Autodesk Fusion 360 part; units mm, degrees
sketch "Sketch1" plane through (0, 0, 0) normal (1, 0, 0) x (0, 1, 0)
  line L0 (0, 0) -> (101.6, 0)
  line L1 (101.6, 0) -> (101.6, 381)
  line L2 (101.6, 381) -> (0, 381)
  line L3 (0, 381) -> (0, 0)
  line L4 (50.8, 381) -> (0, 381)
  line L5 (0, 381) -> (0, 374.65)
  line L6 (0, 374.65) -> (50.8, 374.65)
  line L7 (50.8, 374.65) -> (50.8, 381)
  dimension "d1" = 101.6
  dimension "d2" = 381
  dimension "d3" = 6.35
  dimension "d5" = 50.8
extrude "Extrude1" add sketch "Sketch1" along normal blind 6.35 contours L0 L1 L2 L3 L6 L7
Can you work these out from the model? Positions are in its coordinate system, mm. A direction names the side the tool comes from. Coordinates: 2 decimals unless noted, no trailing zeros. Loops run counter-clockwise (first coordinate to the right, second up) from the corner with the lowest first, then second, coordinate; pieces in that order, holes last. Notation, with made-up numbers: (40, -32.5) - (81, -32.5) arc R27 cw to (81, -16.5) - close; hole circle Ø2 at (-27, -19). An arc over 180 degrees is marked (long way). Answer as CSV lines item,"result". Start each with the question number.
1) Which directions (+Z, -Z, +X, -X, +Y, -Y) give clear straight access to the entire face, cutting with the end or side of a thin tool? Please do faces 1 (the flat face through (3, 50, 0)), 2 (the flat face through (3, 25, 374.65)).
2) For pin 1 (1.9 mm diameter, centred on x = 2.5, y = 20, fed in from +Z); pin 2 (3 mm diameter, centred on x = 2.5, z = 378.5, fed in from -Y), each with a flat end and sliding along its axis, tell me the tip position at first contact or that it passes through.
3) I need wall thicknesses on line 1 (Z direction, x = 5.25, y = 31.5). Which ranges of the line are inside material? Lowest first, please. Write a range as from..to.
4) Suppose I cut it at A-A (y = 19). Please give me the cut outline in (x, z).
Check result:
1,face 1,"-Z, +X, -X, +Y, -Y"
1,face 2,"+Z, +X, -X, -Y"
2,pin 1,"stops at z = 374.65"
2,pin 2,"stops at y = 50.8"
3,line 1,"z = 0..374.65"
4,outline,"(0, 0) - (6.35, 0) - (6.35, 374.65) - (0, 374.65) - close"
